Design review of the part built by this model. Coordinates are the model's own, in mm. Face numbers are marked on the shaded views. A direction names the side the tool comes from. Coordinates: 2 decimals unless noted, no trailing zeros. Loops run counter-clockwise (first coordinate to the right, second up) from the corner with the lowest first, then second, coordinate; pieces in that order, holes last. Notation, with made-up numbers: (28.5, 58.25) - (69.5, 58.25) arc R7 ccw to (69.5, 65.25) - close; hole circle Ø3 at (51.5, 50). An arc over 180 degrees is marked (long way). Return JSON: item names as keys, results as strings. Group by question number.
from build123d import *

# Parameters (mm, degrees)
PAD_DEPTH       = 20
POCKET_DEPTH    = 15
POCKET001_DEPTH = 263.99865
SKETCH014_R     = 4.85
SKETCH014_R_2   = 2.425
SKETCH014_R_3   = 4
POCKET002_DEPTH = 5.001
SKETCH002_W     = 119.3
SKETCH002_H     = 68.7
PAD001_DEPTH    = 1.96
SKETCH003_W     = 109.6
SKETCH003_H     = 61.6
PAD002_DEPTH    = 1


with BuildPart() as part:
    # Sketch → Pad (new body)
    with BuildSketch(Plane.XZ):
        with BuildLine():
            ThreePointArc((-131.99765, 38.055004), (-97.721492, 52.596551), (-67.607356, 74.492906))
            ThreePointArc((67.607356, 74.492906), (0, 100.809493), (-67.607356, 74.492906))
            ThreePointArc((67.607356, 74.492906), (98.150505, 53.35467), (131.99765, 38.055004))
            Line((131.99765, 38.055004), (131.99765, 4.702024))
            Line((131.99765, 4.702024), (-131.99765, 4.702024))
            Line((-131.99765, 4.702024), (-131.99765, 38.055004))
        make_face()
    extrude(amount=PAD_DEPTH)

    # Sketch012 → Pocket (cut)
    with BuildSketch(Plane.XZ.offset(20)):
        with BuildLine():
            Line((-126.99765, -34.311944), (126.99765, -34.311944))
            Line((126.99765, -34.311944), (126.99765, 34.620733))
            ThreePointArc((67.607356, 69.492906), (95.451831, 48.904968), (126.99765, 34.620733))
            ThreePointArc((67.607356, 69.492906), (0, 95.809493), (-67.607356, 69.492906))
            ThreePointArc((-126.99765, 34.620733), (-95.451831, 48.904968), (-67.607356, 69.492906))
            Line((-126.99765, -34.311944), (-126.99765, 34.620733))
        make_face()
    extrude(amount=-POCKET_DEPTH, mode=Mode.SUBTRACT)

    # Sketch013 → Pocket001 (cut, through all)
    with BuildSketch(Plane.YZ.offset(132)):
        with BuildLine():
            Line((-20, 4.702024), (-5, 4.702024))
            Line((-5, 4.702024), (-5, 38.055004))
            ThreePointArc((-5, 38.055004), (-6.952423, 47.67633), (-12.500816, 55.77554))
            ThreePointArc((-20, 74.492906), (-18.05546, 64.411022), (-12.500816, 55.77554))
            Line((-20, 4.702024), (-20, 74.492906))
        make_face()
    extrude(amount=-POCKET001_DEPTH, mode=Mode.SUBTRACT)

    # Sketch014 → Pocket002 (cut, through all)
    with BuildSketch(Plane.XZ.offset(5)):
        with Locations((-50, 14)):
            Circle(SKETCH014_R)
        with Locations((-28, 14)):
            Circle(SKETCH014_R_2)
        with Locations((28, 14)):
            Circle(SKETCH014_R_2)
        with Locations((50, 14)):
            Circle(SKETCH014_R)
        with Locations((-87.350586, 19.199383)):
            Circle(SKETCH014_R_3)
        with Locations((87.350586, 19.199383)):
            Circle(SKETCH014_R_3)
    extrude(amount=-POCKET002_DEPTH, mode=Mode.SUBTRACT)

    # Sketch002 → Pad001 (join)
    with BuildSketch(Plane(origin=(0, -5, 40), x_dir=(1, 0, 0), z_dir=(0, -1, 0))):
        Rectangle(SKETCH002_W, SKETCH002_H)
    extrude(amount=PAD001_DEPTH)

    # Sketch003 → Pad002 (join)
    with BuildSketch(Plane(origin=(0, -6.96, 40), x_dir=(1, 0, 0), z_dir=(0, -1, 0))):
        with Locations((3.15, 0)):
            Rectangle(SKETCH003_W, SKETCH003_H)
    extrude(amount=PAD002_DEPTH)


solid = part.part
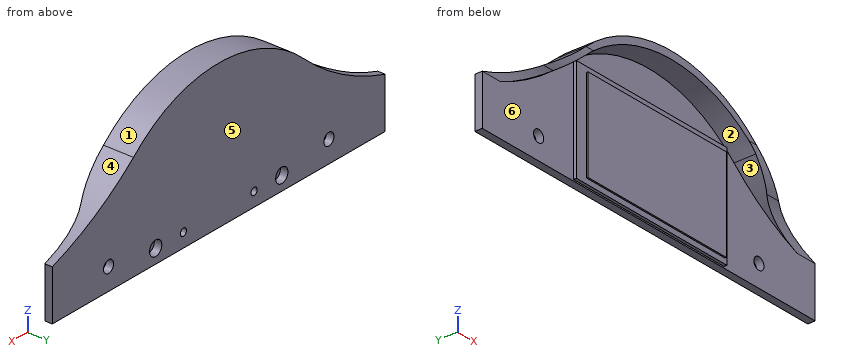
Item 1: Add section C-C (z = 51.5). State the section outline as (x, y) points.
Item 2: For the marked faces 1, 2 and 3, list the 3-axis set-ups (+Z, -Z, +X, -X, +Y, -Y) from which the entire face can be reached by the end or side of a thin tool; tool diameter is ignored.
Item 3: For P1, Ø4, axis at y = -10, z = 67, coming from the +X side; P2, Ø3, axis at x = -18, y = -15, coming from the -Z side; P3, Ø18.5, axis at x = -23.5, z = 54.5, coming from the -Y side, all flat-tipped, find the tip position at first contact; note any pin that passes through.
Item 4: Add section D-D (x = -13). State the section outline as (y, z) points.
Item 5: To check wall thickness, follow line 1 (Y direction, x = -59, z = 37.5); line 2 (Y direction, x = 18, z = 18.5); line 3 (Z direction, x = 28, y = -2.4) (1 decimal). State the ranges of each line that lie inside material, in increasing order. Write a range as from..to.
Item 6: Add section A-A (z = 31). State the section outline as (x, y) points, then the cut area to 3 significant figures.
Item 7: Draft analysis for pull direction X (two halves, no side actions). For the marked faces 4, 5 and 6, state which applies: pulls with the +X half, pulls with the -X half, needs draft (parallel to the pull), parting line crosses it, or undercut.
Answers below:
{
 "1": {"outline": "(-99.69, -8.98) - (-91.18, -8.98) - (-91.18, -5) - (-59.65, -5) - (-59.65, -6.96) - (-51.65, -6.96) - (-51.65, -7.96) - (57.95, -7.96) - (57.95, -6.96) - (59.65, -6.96) - (59.65, -5) - (91.18, -5) - (91.18, -8.98) - (101.5, -8.98) - (101.5, 0) - (-99.69, 0) - close"},
 "2": {"face 1": "+Z, +Y, -Y", "face 2": "-Y", "face 3": "-Z, -Y"},
 "3": {"P1": "stops at x = 79.89", "P2": "stops at z = 93.89", "P3": "stops at y = -7.96"},
 "4": {"outline": "(-20, 94.96) - (-5, 94.96) - (-5, 74.35) - (-6.96, 74.35) - (-6.96, 70.8) - (-7.96, 70.8) - (-7.96, 9.2) - (-6.96, 9.2) - (-6.96, 5.65) - (-5, 5.65) - (-5, 4.7) - (0, 4.7) - (0, 99.96) - (-20, 99.96) - close"},
 "5": {"line 1": "y = -6.96..0", "line 2": "y = -7.96..0", "line 3": "z = 4.7..11.6, 16.4..96.8"},
 "6": {"outline": "(-132, -5) - (-59.65, -5) - (-59.65, -6.96) - (-51.65, -6.96) - (-51.65, -7.96) - (57.95, -7.96) - (57.95, -6.96) - (59.65, -6.96) - (59.65, -5) - (132, -5) - (132, 0) - (-132, 0) - close", "area": "1,660 mm^2"},
 "7": {"face 4": "pulls with the +X half", "face 5": "needs draft", "face 6": "undercut"}
}
